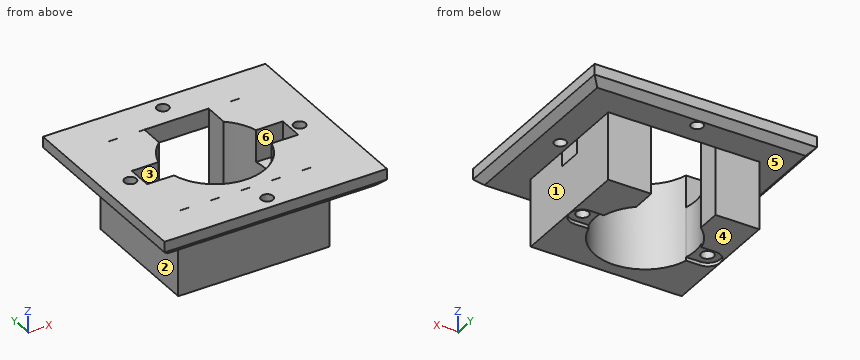
```python
from build123d import *

# Parameters (mm, degrees)
F0_W      = 42.3
F0_H      = 35.2431833744
F0_R      = 1.75
F1_DEPTH  = 20
F3_DEPTH  = 20
F4_DEPTH  = 1
F5_R      = 1.75
F6_DEPTH  = 5
F7_W      = 62.3000003397
F7_H      = 55.2812255919
F8_DEPTH  = 4
F9_DEPTH  = 1
F10_DEPTH = 4
F11_R     = 1.6604727816
F12_DEPTH = 6
F13_SIZE  = 2


with BuildPart() as f1:
    # F0 (on Top) → F1 (new body)
    with BuildSketch(Plane.XY):
        Rectangle(F0_W, F0_H)
        with BuildLine():
            ThreePointArc((-13.6586968632, 3.5), (0, 14.1), (13.6586968632, 3.5))
            Line((13.6586968632, 3.5), (17.6, 3.5))
            ThreePointArc((17.6, 3.5), (20.0748737342, 2.4748737342), (21.1, 0))
            ThreePointArc((21.1, 0), (20.0748737342, -2.4748737342), (17.6, -3.5))
            Line((17.6, -3.5), (13.6586968632, -3.5))
            ThreePointArc((13.6586968632, -3.5), (0, -14.1), (-13.6586968632, -3.5))
            Line((-13.6586968632, -3.5), (-17.6, -3.5))
            ThreePointArc((-17.6, -3.5), (-20.0748737342, -2.4748737342), (-21.1, 0))
            ThreePointArc((-21.1, 0), (-20.0748737342, 2.4748737342), (-17.6, 3.5))
            Line((-17.6, 3.5), (-13.6586968632, 3.5))
        make_face(mode=Mode.SUBTRACT)
        with BuildLine():
            ThreePointArc((-14.1, 0), (-13.9892391818, 1.7638557522), (-13.6586968632, 3.5))
            Line((-13.6586968632, 3.5), (-17.6, 3.5))
            ThreePointArc((-17.6, 3.5), (-20.0748737342, 2.4748737342), (-21.1, 0))
            ThreePointArc((-21.1, 0), (-20.0748737342, -2.4748737342), (-17.6, -3.5))
            Line((-17.6, -3.5), (-13.6586968632, -3.5))
            ThreePointArc((-13.6586968632, -3.5), (-13.9892391818, -1.7638557522), (-14.1, 0))
        make_face()
        with Locations((-17.5, 0)):
            Circle(F0_R, mode=Mode.SUBTRACT)
        with BuildLine():
            ThreePointArc((13.6586968632, 3.5), (13.9892391818, 1.7638557522), (14.1, 0))
            ThreePointArc((14.1, 0), (13.9892391818, -1.7638557522), (13.6586968632, -3.5))
            Line((13.6586968632, -3.5), (17.6, -3.5))
            ThreePointArc((17.6, -3.5), (20.0748737342, -2.4748737342), (21.1, 0))
            ThreePointArc((21.1, 0), (20.0748737342, 2.4748737342), (17.6, 3.5))
            Line((17.6, 3.5), (13.6586968632, 3.5))
        make_face()
        with BuildLine():
            ThreePointArc((19.25, 0), (17.5, -1.75), (15.75, 0))
            ThreePointArc((15.75, 0), (17.5, 1.75), (19.25, 0))
        make_face(mode=Mode.SUBTRACT)
    extrude(amount=F1_DEPTH)

    # F2 (on face) → F3 (cut)
    with BuildSketch(Plane.XY.offset(20)):
        with BuildLine():
            Line((9.1142978397, 17.6215916872), (-8.8857021603, 17.6215916872))
            Line((-8.8857021603, 17.6215916872), (-8.9292200042, 10.9123338529))
            ThreePointArc((-8.9292200042, 10.9123338529), (0.0914540337, 14.0997034068), (9.0700227445, 10.7955864784))
            Line((9.0700227445, 10.7955864784), (9.1142978397, 17.6215916872))
        make_face()
    extrude(amount=-F3_DEPTH, mode=Mode.SUBTRACT)

    # F0 (on Top) → F4 (cut)
    with BuildSketch(Plane.XY):
        with BuildLine():
            ThreePointArc((-14.1, 0), (-13.9892391818, 1.7638557522), (-13.6586968632, 3.5))
            Line((-13.6586968632, 3.5), (-17.6, 3.5))
            ThreePointArc((-17.6, 3.5), (-20.0748737342, 2.4748737342), (-21.1, 0))
            ThreePointArc((-21.1, 0), (-20.0748737342, -2.4748737342), (-17.6, -3.5))
            Line((-17.6, -3.5), (-13.6586968632, -3.5))
            ThreePointArc((-13.6586968632, -3.5), (-13.9892391818, -1.7638557522), (-14.1, 0))
        make_face()
        with Locations((-17.5, 0)):
            Circle(F0_R, mode=Mode.SUBTRACT)
        with BuildLine():
            ThreePointArc((13.6586968632, 3.5), (13.9892391818, 1.7638557522), (14.1, 0))
            ThreePointArc((14.1, 0), (13.9892391818, -1.7638557522), (13.6586968632, -3.5))
            Line((13.6586968632, -3.5), (17.6, -3.5))
            ThreePointArc((17.6, -3.5), (20.0748737342, -2.4748737342), (21.1, 0))
            ThreePointArc((21.1, 0), (20.0748737342, 2.4748737342), (17.6, 3.5))
            Line((17.6, 3.5), (13.6586968632, 3.5))
        make_face()
        with BuildLine():
            ThreePointArc((19.25, 0), (17.5, -1.75), (15.75, 0))
            ThreePointArc((15.75, 0), (17.5, 1.75), (19.25, 0))
        make_face(mode=Mode.SUBTRACT)
    extrude(amount=F4_DEPTH, mode=Mode.SUBTRACT)

    # F5 (on face) → F6 (cut)
    with BuildSketch(Plane.XY.offset(20)):
        with BuildLine():
            ThreePointArc((-13.6586968632, -3.5), (-14.1, 0), (-13.6586968632, 3.5))
            Line((-13.6586968632, 3.5), (-21.15, 3.5))
            Line((-21.15, 3.5), (-21.15, -3.5))
            Line((-21.15, -3.5), (-13.6586968632, -3.5))
        make_face()
        with Locations((-17.5, 0)):
            Circle(F5_R, mode=Mode.SUBTRACT)
        with BuildLine():
            Line((21.15, -3.5), (21.15, 3.5))
            Line((21.15, 3.5), (13.6586968632, 3.5))
            ThreePointArc((13.6586968632, 3.5), (14.1, 0), (13.6586968632, -3.5))
            Line((13.6586968632, -3.5), (21.15, -3.5))
        make_face()
        with Locations((17.5, 0)):
            Circle(F5_R, mode=Mode.SUBTRACT)
    extrude(amount=-F6_DEPTH, mode=Mode.SUBTRACT)

    # F10 (add): faces of the model
    f10_faces = [f1.faces().sort_by_distance(p)[0] for p in [
        (-15.655980784, 11.1858977237, 20),
        (15.7115170965, 11.1581962094, 20),
        (-20.704050524, -10.5607958436, 20),
    ]]


with BuildPart() as f8:
    # F7 (on face) → F8 (new body)
    with BuildSketch(Plane.XY.offset(20)):
        Rectangle(F7_W, F7_H)
        Polygon((-21.15, 17.6406126261), (21.15, 17.6406126261), (21.15, -17.6406126261), (-21.15, -17.6406126261), (-21.15, 3.5), (-21.15, 17.6215916872), align=None, mode=Mode.SUBTRACT)
    extrude(amount=F8_DEPTH)


with BuildPart() as f9:
    # F9 (new): a face of the model
    f9_faces = [f8.part.faces().sort_by_distance(p)[0] for p in [
        (0, -26.8077080028, 20),
    ]]
    extrude(f9_faces, amount=F9_DEPTH)


with BuildPart() as f1_1:
    add(f1.part)

    add(f8.part)  # F10 merges F8

    add(f9.part)  # F10 merges F9
    extrude(f10_faces, amount=F10_DEPTH)

    # F11 (on face) → F12 (cut)
    with BuildSketch(Plane(origin=(0, 0, 19), x_dir=(1, 0, 0), z_dir=(0, 0, -1))):
        with Locations((0, 23.7122699618)):
            Circle(F11_R)
        with Locations((23.7122699618, 0)):
            Circle(F11_R)
        with Locations((0, -23.7122699618)):
            Circle(F11_R)
        with Locations((-23.7122699618, 0)):
            Circle(F11_R)
    extrude(amount=-F12_DEPTH, mode=Mode.SUBTRACT)

    # F13
    f13_edges = [f1_1.edges().sort_by_distance(p)[0] for p in [
        (-31.15, 0, 19),
        (0, -27.640613, 19),
        (31.15, 0, 19),
        (0, 27.640613, 19),
    ]]
    chamfer(f13_edges, length=F13_SIZE)


solid = f1_1.part
```
Geometry: final body of the model. Coordinates: model frame, mm. Face numbers are marked on the shaded views. A direction names the side the tool comes from. Round coordinates to 2 decimals unless told otherwise and drop trailing zeros. Write each loop counter-clockwise with the first axis right and the second up, starting at its lowest first coordinate (ties: lowest second). Pieces come first, ordered by that corner, then holes.
Item 1: Material intervals for L1, parallel to X at y = 15, z = 4.5; L2, parallel to Y at x = -17.5, z = 6; L3, parallel to Z at x = 26, y = -13, sorted ascending.
Item 2: Section query D-D (x = 0). Return loops of the section in (y, z), plus the area to 3 significant figures.
Item 3: Pin query (flat end, axial travel): P1, Ø5, axis at x = -1.5, z = 11.5, coming from the +Y side; P2, Ø10, axis at x = -17, z = 10, coming from the +Y side; P3, Ø8, axis at x = -2, y = -7.5, coming from the -Z side; P4, Ø9.5, axis at y = 1, z = 8, coming from the +X side. Return the tip coordinate at first contact, or that it passes through.
Item 4: Section query A-A (x = -15). Return loops of the section in (y, z).
Item 5: Mould query, pull axis X, two halves, no side actions, for the marked faces 1, 2 and 3. Classes: +X half, -X half, draft (parallel to the pull), parting line (faces both ways), or undercut.
Item 6: Set-up query: the marked faces 4, 5 and 6. Return all of +Z, -Z, +X, -X, +Y, -Y with unobstructed straight access to the full face (end or side cutting, diameter ignored); none if empty.
Item 7: Section query B-B (z = 16.25). Return loops of the section in (x, y).
Item 8: Section query C-C (y = -5). Return loops of the section in (x, z), plus the area to 3 significant figures.
Completed:
1. L1: x = -21.15 to -8.9, 9.1 to 21.15
1. L2: y = -17.62 to -1.75, 1.75 to 17.62
1. L3: z = 19 to 24
2. outline: (-27.64, 21) - (-25.64, 19) - (-25.37, 19) - (-25.37, 24) - (-27.64, 24) - close; (-22.05, 19) - (-17.64, 19) - (-17.64, 24) - (-22.05, 24) - close; (-17.62, 0) - (-14.1, 0) - (-14.1, 24) - (-17.62, 24) - close; (17.64, 19) - (22.05, 19) - (22.05, 24) - (17.64, 24) - close; (25.37, 19) - (25.64, 19) - (27.64, 21) - (27.64, 24) - (25.37, 24) - close
2. area: 147 mm2
3. P1: stops at y = -13.52
3. P2: stops at y = 17.62
3. P3: passes through
3. P4: stops at x = 21.15
4. outline: (-27.64, 21) - (-25.64, 19) - (-17.64, 19) - (-17.64, 24) - (-27.64, 24) - close; (-17.62, 0) - (-3.5, 0) - (-3.5, 1) - (3.5, 1) - (3.5, 0) - (17.62, 0) - (17.62, 24) - (3.5, 24) - (3.5, 15) - (-3.5, 15) - (-3.5, 24) - (-17.62, 24) - close; (17.64, 19) - (25.64, 19) - (27.64, 21) - (27.64, 24) - (17.64, 24) - close
5. face 1: +X half
5. face 2: -X half
5. face 3: undercut
6. face 4: -Z, +X, -X, +Y, -Y
6. face 5: -Z
6. face 6: +Z
7. outline: (-21.15, -17.62) - (21.15, -17.62) - (21.15, -3.5) - (13.66, -3.5) arc R14.1 cw to (-13.66, -3.5) - (-21.15, -3.5) - close; (-21.15, 3.5) - (-13.66, 3.5) arc R14.1 cw to (-8.93, 10.91) - (-8.89, 17.62) - (-21.15, 17.62) - close; (9.07, 10.8) arc R14.1 cw to (13.66, 3.5) - (21.15, 3.5) - (21.15, 17.62) - (9.11, 17.62) - close
8. outline: (-31.15, 21) - (-29.15, 19) - (-21.15, 19) - (-21.15, 0) - (-13.18, 0) - (-13.18, 24) - (-31.15, 24) - close; (13.18, 0) - (21.15, 0) - (21.15, 19) - (29.15, 19) - (31.15, 21) - (31.15, 24) - (13.18, 24) - close
8. area: 478 mm2
